Check sheet for the modelled part. Datum: model origin and axes. Units: mm. Face numbers are marked on the shaded views. Give positions to 0.01 mm unless a question says otherwise; leave off trailing zeros. Write each loop counter-clockwise with the first axis right and the second up, starting at its lowest first coordinate (ties: lowest second). Pieces come first, ordered by that corner, then holes. Notation, with made-up numbers: (35, 67.5) - (60, 67.5) arc R21 ccw to (60, 86.5) - close; hole circle Ø3 at (-24, 75.5). An arc over 180 degrees is marked (long way). Return JSON: item names as keys, results as strings. Group by question number.
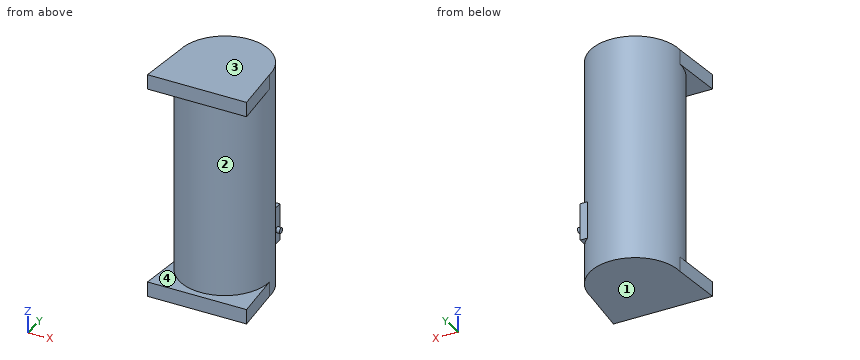
```python
from build123d import *

# Parameters (mm, degrees)
SKETCH1_R           = 60.72
BOSS_EXTRUDE1_DEPTH = 308.6
BOSS_EXTRUDE2_DEPTH = 20
BOSS_EXTRUDE3_DEPTH = 20
SKETCH4_W           = 50.6
SKETCH4_H           = 12.7
BOSS_EXTRUDE4_DEPTH = 20
SKETCH5_R           = 3.8
BOSS_EXTRUDE5_DEPTH = 5


with BuildPart() as part:
    # Sketch1 → Boss-Extrude1 (new body)
    with BuildSketch(Plane.XY):
        Circle(SKETCH1_R)
    extrude(amount=BOSS_EXTRUDE1_DEPTH)

    # Sketch2 → Boss-Extrude2 (add)
    with BuildSketch(Plane.XY.offset(308.6)):
        Polygon((67.3, -69.512383737), (-67.3, -69.512383737), (-60.72, 0), (60.72, 0), align=None)
    extrude(amount=-BOSS_EXTRUDE2_DEPTH)

    # Sketch3 → Boss-Extrude3 (add)
    with BuildSketch(Plane(origin=(0, 0, 0), x_dir=(-1, 0, 0), z_dir=(0, 0, -1))):
        Polygon((2.236970423, -69.512383737), (-67.3, -69.512383737), (-60.72, 0), (60.72, 0), (67.3, -69.512383737), align=None)
    extrude(amount=-BOSS_EXTRUDE3_DEPTH)

    # Sketch4 → Boss-Extrude4 (add)
    with BuildSketch(Plane(origin=(50, 0, 0), x_dir=(0, 0, -1), z_dir=(1, 0, 0))):
        with Locations((-76.3, 39.37)):
            Rectangle(SKETCH4_W, SKETCH4_H)
    extrude(amount=-BOSS_EXTRUDE4_DEPTH)

    # Sketch5 → Boss-Extrude5 (add)
    with BuildSketch(Plane(origin=(50, 0, 0), x_dir=(0, 0, -1), z_dir=(1, 0, 0))):
        with Locations((-69, 39.37)):
            Circle(SKETCH5_R)
    extrude(amount=BOSS_EXTRUDE5_DEPTH)


solid = part.part
```
Item 1: Section check D-D on z = 247.5. Record the cut outline in (x, y), plus the area to 3 significant figures.
Item 2: Depth check by flat-ended pin: pin 1 (6 mm diameter, centred on x = 9.5, z = 62.5, fed in from +Y); pin 2 (6 mm diameter, centred on x = -50.5, z = 191, fed in from -Y); pin 3 (8 mm diameter, centred on x = 42.5, z = 85, fed in from +Y); pin 4 (11 mm diameter, centred on x = 47.5, y = 39.5, fed in from -Z). Enter the tip coordinate at first touch or a pass-through.
Item 3: Material ranges on line 1 along Z through (x, y) = (-54, -40.5); line 2 along Y through (x, z) = (1, 131); line 3 along X through (y, z) = (-34, 72), recorded low to high. Write a range as from..to.
Item 4: Section check A-A on z = 69. Record the cut outline in (x, y), plus the area to 3 significant figures.
Item 5: Section check C-C on y = 39.37. Record the cut outline in (x, z).
Item 6: Mould release check, pull along Z, two halves, no side actions. Record for the marked faces 1, 2, 3 and 4: +Z half, -Z half, draft (parallel to the pull), parting line (faces both ways), or undercut.
Item 7: Section check B-B on x = 0. Record the cut outline in (y, z), plus the area to 3 significant figures.
Reply:
{
 "1": {"outline": "circle Ø121.44 at (0, 0)", "area": "11,600 mm²"},
 "2": {"pin 1": "y = 60.37", "pin 2": "y = -37.82", "pin 3": "y = 46.95", "pin 4": "z = 0"},
 "3": {"line 1": "0..20, 288.6..308.6", "line 2": "-60.71..60.71", "line 3": "-50.31..50.31"},
 "4": {"outline": "(39.96, 45.72) arc R60.72 ccw (long way) to (50, 34.45) - (50, 35.57) - (55, 35.57) - (55, 43.17) - (50, 43.17) - (50, 45.72) - close", "area": "11,700 mm²"},
 "5": {"outline": "(-46.23, 0) - (46.23, 0) - (46.23, 51) - (50, 51) - (50, 65.2) - (55, 65.2) - (55, 72.8) - (50, 72.8) - (50, 101.6) - (46.23, 101.6) - (46.23, 308.6) - (-46.23, 308.6) - close"},
 "6": {"face 1": "-Z half", "face 2": "undercut", "face 3": "+Z half", "face 4": "undercut"},
 "7": {"outline": "(-69.51, 0) - (60.72, 0) - (60.72, 308.6) - (-69.51, 308.6) - (-69.51, 288.6) - (-60.72, 288.6) - (-60.72, 20) - (-69.51, 20) - close", "area": "37,800 mm²"}
}
